from build123d import *

# Parameters (mm, degrees)
SKETCH1_R           = 21.59
SKETCH1_R_2         = 9.144
BOSS_EXTRUDE1_DEPTH = 70.1
SKETCH2_R           = 16.4084
SKETCH2_R_2         = 16.256
BOSS_EXTRUDE2_DEPTH = 38.1


with BuildPart() as part:
    # Sketch1 → Boss-Extrude1 (new body)
    with BuildSketch(Plane.XY):
        Circle(SKETCH1_R)
        with Locations((0.118855304, -11.557)):
            Circle(SKETCH1_R_2, mode=Mode.SUBTRACT)
        with Locations((9.955579479, 5.869470694)):
            Circle(SKETCH1_R_2, mode=Mode.SUBTRACT)
        with Locations((-10.060900468, 5.687049391)):
            Circle(SKETCH1_R_2, mode=Mode.SUBTRACT)
    extrude(amount=BOSS_EXTRUDE1_DEPTH)

    # Sketch2 → Boss-Extrude2 (add)
    with BuildSketch(Plane.XY.offset(70.1)):
        Circle(SKETCH2_R)
        Circle(SKETCH2_R_2, mode=Mode.SUBTRACT)
    extrude(amount=BOSS_EXTRUDE2_DEPTH)

    # Sketch8 → Revolve3 (revolve)
    with BuildSketch(Plane(origin=(0, 0, 0), x_dir=(0, 0, -1), z_dir=(1, 0, 0))):
        Polygon((-70.1, 21.56234654), (-82.8, 16.4084), (-70.1, 16.4084), align=None)
    revolve(axis=Axis((0, 0, 126.159811209), (0, 0, -1)))


solid = part.part
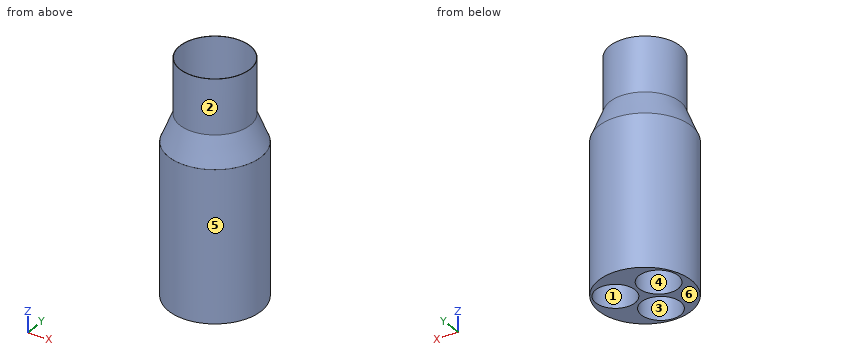
Verification items for the finished model (mm, model axes). Face numbers are marked on the shaded views. A direction names the side the tool comes from. Give positions to 0.01 mm unless a question says otherwise; leave off trailing zeros. Order: outer loops, then holes, each group sorted by start corner. A loop starts at its lowest first (then second) coordinate and runs counter-clockwise, first axis right, second up. Notation, with made-up numbers: M 82,1.5 L 120,1.5 A15 cw 120,23.5 Z; hole C 75,-1 d7. An arc over 180 degrees is marked long. Answer as a JSON object with one key per item and string values. Group by question number.
1) Cross-section at D-D (z = 36). Enter the section's corners in (x, y), then the cut area to 3 significant figures.
2) Cross-section at A-A (y = 7). Give the number of separate pieces and of enclosed holes in the cut face, then the cut area to 3 significant figures.
3) Depth check by flat-ended pin: pin 1 Ø2 at (x, z) = (-7, 32.5) entering from -Y; pin 2 Ø8 at (x, y) = (2, -16) entering from -Z; pin 3 Ø12 at (y, z) = (-13, 20) entering from +X. Enter the tip coordinate at first touch or a pass-through.
4) Scan lines: line 1 along Y through (x, z) = (0.5, 97.5); line 2 along X through (y, z) = (0, 93.5); line 3 along X through (y, z) = (10.5, 14). Record each from-to range of solid material in increasing order. Write a range as [from, to].
5) Mould release check, pull along X, two halves, no side actions. Record for the marked faces 3, 4, 5 and 6: released by +X, released by -X, zero draft, split by the parting line, or undercut.
6) Access from +Z, -Z, +X, -X, +Y, -Y to the whole of each face (thin tool, end or side, straight path). Record for the marked faces 1 and 2.
7) Cross-section at B-B (z = 94.5). Enter the section's corners in (x, y).
Result sheet:
{
 "1": {"outline": "C 0,0 d43.18; hole C -10.06,5.69 d18.29; hole C 0.12,-11.56 d18.29; hole C 9.96,5.87 d18.29", "area": "676 mm2"},
 "2": {"separate pieces": "3", "enclosed holes": "0", "area": "406 mm2"},
 "3": {"pin 1": "stops at y = -20.74", "pin 2": "stops at z = 70.1", "pin 3": "stops at x = 20.42"},
 "4": {"line 1": "y = [-16.4, -16.25], [16.25, 16.4]", "line 2": "x = [-16.41, -16.26], [16.26, 16.41]", "line 3": "x = [-18.86, -17.84], [-2.29, 2.07], [17.84, 18.86]"},
 "5": {"face 3": "undercut", "face 4": "undercut", "face 5": "split by the parting line", "face 6": "zero draft"},
 "6": {"face 1": "-Z", "face 2": "+Z"},
 "7": {"outline": "C 0,0 d32.82; hole C 0,0 d32.51"}
}
